from build123d import *

# Parameters (mm, degrees)
BASE_DEPTH                 = 24.7
DINRAILLEG_START           = -24.7
DINRAILLEG_DEPTH           = 49.4
MAINRIB_START              = -24.7
MAINRIBS_W                 = 2.6
MAINRIBS_H                 = 41.5
MAINRIB_DEPTH              = 49.4
TOPBASE_START              = -24.7
TOPBASES_W                 = 60
TOPBASES_H                 = 2.4
TOPBASE_DEPTH              = 49.4
RIB1_START                 = -24.7
RIB1S_W                    = 50
RIB1S_H                    = 1.2
RIB1_DEPTH                 = 49.4
RIB2_START                 = -24.7
RIB2S_W                    = 46
RIB2S_H                    = 1.2
RIB2_DEPTH                 = 49.4
RIB3_START                 = -24.7
RIB3S_W                    = 40
RIB3S_H                    = 1
RIB3_DEPTH                 = 49.4
RIB4_START                 = -24.7
RIB4S_W                    = 34
RIB4S_H                    = 1
RIB4_DEPTH                 = 49.4
MOUNTINGSLOT_DEPTH         = 68.186977905
M4X0_7_TAPPED_HOLE1_REACH  = 70.267
M4X0_7_TAPPED_HOLE1_BORE_R = 1.65
TBF_R                      = 1
MRF_R                      = 1
FILLET_F1_R                = 0.6
FILLET_F2_R                = 0.6
FILLET_F3_R                = 0.5
FILLET_F4_R                = 0.5


with BuildPart() as part:
    # BaseS → Base (new, symmetric)
    with BuildSketch(Plane(origin=(0, 0, 0), x_dir=(0, 0, -1), z_dir=(1, 0, 0))):
        Polygon((40, -6.5), (30, -6.5), (30, 0), (-30, 0), (-30, -6.5), (-40, -6.5), (-40, -8), (-28.5, -8), (-28.5, -1.5), (28.5, -1.5), (28.5, -8), (40, -8), align=None)
    extrude(amount=BASE_DEPTH, both=True)

    # DinRailLegS → DinRailLeg (add)
    with BuildSketch(Plane(origin=(0, 0, 0), x_dir=(0, 0, -1), z_dir=(1, 0, 0)).offset(DINRAILLEG_START)):
        Polygon((18, -1.5), (18, -5.3), (15, -5.3), (15, -3.8), (16.5, -3.8), (16.5, -1.5), align=None)
    dinrailleg = extrude(amount=DINRAILLEG_DEPTH)

    # MainRibS → MainRib (add)
    with BuildSketch(Plane(origin=(0, 0, 0), x_dir=(0, 0, -1), z_dir=(1, 0, 0)).offset(MAINRIB_START)):
        with Locations((0, 20.75)):
            Rectangle(MAINRIBS_W, MAINRIBS_H)
    extrude(amount=MAINRIB_DEPTH)

    # TopBaseS → TopBase (add)
    with BuildSketch(Plane(origin=(0, 0, 0), x_dir=(0, 0, -1), z_dir=(1, 0, 0)).offset(TOPBASE_START)):
        with Locations((0, 40.3)):
            Rectangle(TOPBASES_W, TOPBASES_H)
    extrude(amount=TOPBASE_DEPTH)

    # Rib1S → Rib1 (add)
    with BuildSketch(Plane(origin=(0, 0, 0), x_dir=(0, 0, -1), z_dir=(1, 0, 0)).offset(RIB1_START)):
        with Locations((0, 31)):
            Rectangle(RIB1S_W, RIB1S_H)
    extrude(amount=RIB1_DEPTH)

    # Rib2S → Rib2 (add)
    with BuildSketch(Plane(origin=(0, 0, 0), x_dir=(0, 0, -1), z_dir=(1, 0, 0)).offset(RIB2_START)):
        with Locations((0, 23.3)):
            Rectangle(RIB2S_W, RIB2S_H)
    extrude(amount=RIB2_DEPTH)

    # Rib3S → Rib3 (add)
    with BuildSketch(Plane(origin=(0, 0, 0), x_dir=(0, 0, -1), z_dir=(1, 0, 0)).offset(RIB3_START)):
        with Locations((0, 15.7)):
            Rectangle(RIB3S_W, RIB3S_H)
    extrude(amount=RIB3_DEPTH)

    # Rib4S → Rib4 (add)
    with BuildSketch(Plane(origin=(0, 0, 0), x_dir=(0, 0, -1), z_dir=(1, 0, 0)).offset(RIB4_START)):
        with Locations((0, 8.2)):
            Rectangle(RIB4S_W, RIB4S_H)
    extrude(amount=RIB4_DEPTH)

    # MountingSlotS → MountingSlot (cut, through all)
    with BuildSketch(Plane(origin=(0, -6.5, 0), x_dir=(1, 0, 0), z_dir=(0, 1, 0))):
        with BuildLine():
            Line((2.7, 40), (2.7, 34))
            ThreePointArc((2.7, 34), (0, 31.3), (-2.7, 34))
            Line((-2.7, 34), (-2.7, 40))
            ThreePointArc((-2.7, 40), (0, 42.7), (2.7, 40))
        make_face()
    mountingslot = extrude(amount=-MOUNTINGSLOT_DEPTH, mode=Mode.SUBTRACT)

    # M4x0.7 Tapped Hole1 bore → M4x0.7 Tapped Hole1 (cut, up to next)
    with BuildSketch(Plane(origin=(0, 41.5, 0), x_dir=(1, 0, 0), z_dir=(0, 1, 0)), mode=Mode.PRIVATE) as m4x0_7_tapped_hole1_sk1:
        with Locations((0, 24)):
            Circle(M4X0_7_TAPPED_HOLE1_BORE_R)
    m4x0_7_tapped_hole1_tool1 = extrude(m4x0_7_tapped_hole1_sk1.sketch, amount=-M4X0_7_TAPPED_HOLE1_REACH, mode=Mode.PRIVATE) & part.part
    m4x0_7_tapped_hole1 = m4x0_7_tapped_hole1_tool1.solids().sort_by_distance((0, 41.5, -24))[0]
    add(m4x0_7_tapped_hole1, mode=Mode.SUBTRACT)

    # Mounting Features VM: DinRailLeg, MountingSlot, M4x0.7 Tapped Hole1 across plane
    add(dinrailleg.mirror(Plane.XY))
    add(mountingslot.mirror(Plane.XY), mode=Mode.SUBTRACT)
    add(m4x0_7_tapped_hole1.mirror(Plane.XY), mode=Mode.SUBTRACT)

    # TBF
    tbf_edges = [part.edges().sort_by_distance(p)[0] for p in [
        (0, 41.5, -30),
        (0, 39.1, 30),
        (0, 39.1, -30),
        (0, 41.5, 30),
    ]]
    fillet(tbf_edges, radius=TBF_R)

    # MRF
    mrf_edges = [part.edges().sort_by_distance(p)[0] for p in [
        (0, 23.9, -1.3),
        (0, 22.7, -1.3),
        (0, 22.7, 1.3),
        (0, 23.9, 1.3),
        (0, 15.2, -1.3),
        (0, 15.2, 1.3),
        (0, 16.2, -1.3),
        (0, 16.2, 1.3),
        (0, 7.7, -1.3),
        (0, 7.7, 1.3),
        (0, 8.7, -1.3),
        (0, 8.7, 1.3),
        (0, 0, -1.3),
        (0, 0, 1.3),
        (0, 39.1, 1.3),
        (0, 39.1, -1.3),
        (0, 31.6, -1.3),
        (0, 31.6, 1.3),
        (0, 30.4, -1.3),
        (0, 30.4, 1.3),
    ]]
    fillet(mrf_edges, radius=MRF_R)

    # Fillet F1
    fillet_f1_edges = [part.edges().sort_by_distance(p)[0] for p in [
        (0, 30.4, -25),
        (0, 31.6, -25),
        (0, 30.4, 25),
        (0, 31.6, 25),
    ]]
    fillet(fillet_f1_edges, radius=FILLET_F1_R - 0.0001)  # a hair under: the kernel refuses the full size

    # Fillet F2
    fillet_f2_edges = [part.edges().sort_by_distance(p)[0] for p in [
        (0, 23.9, -23),
        (0, 22.7, -23),
        (0, 23.9, 23),
        (0, 22.7, 23),
    ]]
    fillet(fillet_f2_edges, radius=FILLET_F2_R - 0.0001)  # a hair under: the kernel refuses the full size

    # Fillet F3
    fillet_f3_edges = [part.edges().sort_by_distance(p)[0] for p in [
        (0, 15.2, -20),
        (0, 16.2, -20),
        (0, 15.2, 20),
        (0, 16.2, 20),
    ]]
    fillet(fillet_f3_edges, radius=FILLET_F3_R - 0.0001)  # a hair under: the kernel refuses the full size

    # Fillet F4
    fillet_f4_edges = [part.edges().sort_by_distance(p)[0] for p in [
        (0, 8.7, 17),
        (0, 7.7, 17),
        (0, 7.7, -17),
        (0, 8.7, -17),
    ]]
    fillet(fillet_f4_edges, radius=FILLET_F4_R - 0.0001)  # a hair under: the kernel refuses the full size


solid = part.part
Design review of the part built by this model. Coordinates are the model's own, in mm. A direction names the side the tool comes from. Round coordinates to 2 decimals unless told otherwise and drop trailing zeros. Write each loop counter-clockwise with the first axis right and the second up, starting at its lowest first coordinate (ties: lowest second). Pieces come first, ordered by that corner, then holes. Notation, with made-up numbers: M 18.25,87.5 L 77.25,87.5 A12 ccw 77.25,106.5 Z; hole C 79.5,74.25 d6. An arc over 180 degrees is marked long. One line per item, written item: value. Start each with the question number.
1. For faces 1 (the face through (0.3, -6.5, 30.5)), 2 (the face through (0, -3, -16.5)), 3 (the face through (0, 35, -1.3)), 4 (the face through (0, 41.5, 0)), 5 (the face through (0, 35, 1.3)), list the 3-axis set-ups (+Z, -Z, +X, -X, +Y, -Y) from which the entire face can be reached by the end or side of a thin tool; tool diameter is ignored.
2. Clearance check with flat-ended pins moving along their axes: P1, Ø1.6, axis at x = -4, y = -4.5, coming from the +Z side; P2, Ø5, axis at x = 1.5, y = 23.5, coming from the -Z side; P3, Ø4.5, axis at x = 6.5, y = 4, coming from the +Z side. State where each tip first meets the part, or that it passes through.
3. Take a section at B-B on x = 0. State how many separate pieces and enclosed holes the cut face has, then the cut area to 3 significant figures.
4. To check wall thickness, follow probe 1 along Y at (x, z) = (4, 3.5); probe 2 along Z at (x, y) = (0, 40); probe 3 along Z at (x, y) = (12, -4.5). State the ranges of each line that lie inside material, in increasing order. Write a range as from..to.
5. Take a section at A-A on z = -5.5. State the section outline as (x, y) points, then the cut area to 3 significant figures.
6. Draft analysis for pull direction Z (two halves, no side actions). For faces 6 (the face through (0, -1.5, -23)), 7 (the face through (0, 4, -1.3)), 8 (the face through (0, 7.7, 9)), 9 (the face through (0, -3, 18)), state which applies: pulls with the +Z half, pulls with the -Z half, needs draft (parallel to the pull), parting line crosses it, or undercut.
Computed:
1. face 1: +Z, +X, -X, +Y
1. face 2: +X, -X
1. face 3: -Z, +X, -X
1. face 4: +Z, -Z, +X, -X, +Y
1. face 5: +Z, +X, -X
2. P1: stops at z = 30
2. P2: stops at z = -23
2. P3: stops at z = 1.3
3. separate pieces: 3
3. enclosed holes: 0
3. area: 539 mm²
4. probe 1: y = -1.5..0, 7.7..8.7, 15.2..16.2, 22.7..23.9, 30.4..31.6, 39.1..41.5
4. probe 2: z = -29.99..-25.65, -22.35..22.35, 25.65..29.99
4. probe 3: z = -30..-28.5, -18..-15, 15..18, 28.5..30
5. outline: M -24.7,-1.5 L 24.7,-1.5 L 24.7,0 L -24.7,0 Z; M -24.7,7.7 L 24.7,7.7 L 24.7,8.7 L -24.7,8.7 Z; M -24.7,15.2 L 24.7,15.2 L 24.7,16.2 L -24.7,16.2 Z; M -24.7,22.7 L 24.7,22.7 L 24.7,23.9 L -24.7,23.9 Z; M -24.7,30.4 L 24.7,30.4 L 24.7,31.6 L -24.7,31.6 Z; M -24.7,39.1 L 24.7,39.1 L 24.7,41.5 L -24.7,41.5 Z
5. area: 410 mm²
6. face 6: undercut
6. face 7: pulls with the -Z half
6. face 8: needs draft
6. face 9: undercut
